from build123d import *

# Parameters (mm, degrees)
SKETCH2_W           = 140
SKETCH2_H           = 140
SKETCH2_R           = 1.6
SKETCH2_R_2         = 1.4
BOSS_EXTRUDE2_DEPTH = 3
SKETCH3_W           = 16
SKETCH3_H           = 3
SKETCH3_W_2         = 3
SKETCH3_H_2         = 16
CUT_EXTRUDE2_DEPTH  = 3


with BuildPart() as part:
    # Sketch2 → Boss-Extrude2 (new body)
    with BuildSketch(Plane(origin=(0, 0, 0), x_dir=(1, 0, 0), z_dir=(0, 1, 0))):
        Rectangle(SKETCH2_W, SKETCH2_H)
        with Locations(Location((-17.011581703, 44.949159058, 0), (0, 0, 270))):
            Circle(SKETCH2_R, mode=Mode.SUBTRACT)
        with Locations(Location((-18.611581703, -3.350840942, 0), (0, 0, 270))):
            Circle(SKETCH2_R, mode=Mode.SUBTRACT)
        with Locations(Location((33.788418297, 29.649159058, 0), (0, 0, 270))):
            Circle(SKETCH2_R, mode=Mode.SUBTRACT)
        with Locations(Location((33.788418297, 1.749159058, 0), (0, 0, 270))):
            Circle(SKETCH2_R, mode=Mode.SUBTRACT)
        with Locations(Location((0, 60, 0), (0, 0, 270))):
            Circle(SKETCH2_R, mode=Mode.SUBTRACT)
        with Locations(Location((-60, 0, 0), (0, 0, 270))):
            Circle(SKETCH2_R, mode=Mode.SUBTRACT)
        with Locations(Location((0, -60, 0), (0, 0, 270))):
            Circle(SKETCH2_R, mode=Mode.SUBTRACT)
        with Locations(Location((60, 0, 0), (0, 0, 270))):
            Circle(SKETCH2_R, mode=Mode.SUBTRACT)
        with Locations(Location((-45, 60, 0), (0, 0, 270))):
            Circle(SKETCH2_R, mode=Mode.SUBTRACT)
        with Locations(Location((45, 60, 0), (0, 0, 270))):
            Circle(SKETCH2_R, mode=Mode.SUBTRACT)
        with Locations(Location((-45, -60, 0), (0, 0, 270))):
            Circle(SKETCH2_R, mode=Mode.SUBTRACT)
        with Locations(Location((45, -60, 0), (0, 0, 270))):
            Circle(SKETCH2_R, mode=Mode.SUBTRACT)
        with Locations(Location((-0.030225379, -18.62367845, 0), (0, 0, 270))):
            Circle(SKETCH2_R_2, mode=Mode.SUBTRACT)
        with Locations(Location((-13.780225379, -40.12367845, 0), (0, 0, 270))):
            Circle(SKETCH2_R_2, mode=Mode.SUBTRACT)
        with Locations(Location((13.719774621, -40.12367845, 0), (0, 0, 270))):
            Circle(SKETCH2_R_2, mode=Mode.SUBTRACT)
    extrude(amount=BOSS_EXTRUDE2_DEPTH)

    # Sketch3 → Cut-Extrude2 (cut)
    with BuildSketch(Plane(origin=(0, 3, 0), x_dir=(1, 0, 0), z_dir=(0, 1, 0))):
        with Locations((-22.5, 68.5)):
            Rectangle(SKETCH3_W, SKETCH3_H)
        with Locations((-22.5, -68.5)):
            Rectangle(SKETCH3_W, SKETCH3_H)
        with Locations((22.5, -68.5)):
            Rectangle(SKETCH3_W, SKETCH3_H)
        with Locations((22.5, 68.5)):
            Rectangle(SKETCH3_W, SKETCH3_H)
        with Locations((-68.5, 22.5)):
            Rectangle(SKETCH3_W_2, SKETCH3_H_2)
        with Locations((68.5, 22.5)):
            Rectangle(SKETCH3_W_2, SKETCH3_H_2)
        with Locations((68.5, -22.5)):
            Rectangle(SKETCH3_W_2, SKETCH3_H_2)
        with Locations((-68.5, -22.5)):
            Rectangle(SKETCH3_W_2, SKETCH3_H_2)
    extrude(amount=-CUT_EXTRUDE2_DEPTH, mode=Mode.SUBTRACT)


solid = part.part
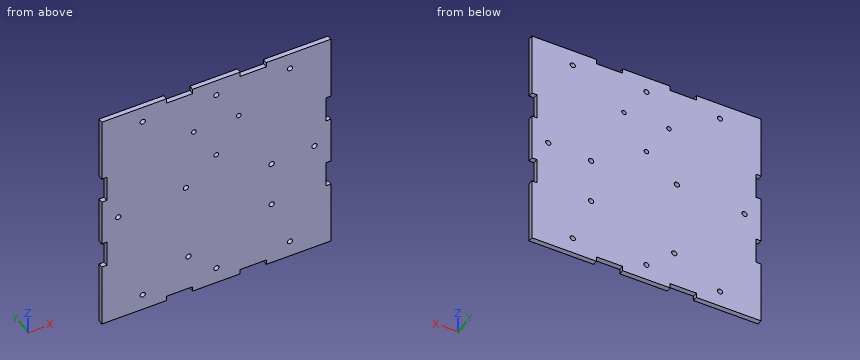
Can you work these out from the model? Positions are in its coordinate system, mm. Coordinates: 2 decimals unless noted, no trailing zeros. Order: outer loops, then holes, each group sorted by start corner. A loop starts at its lowest first (then second) coordinate and runs counter-clockwise, first axis right, second up. Notation, with made-up numbers: (2.5, 3.5) - (46.5, 3.5) arc R20 ccw to (46.5, 23.5) - close; hole circle Ø7 at (-5, 85). An arc over 180 degrees is marked (long way). Answer as a JSON object with one key per item and string values. Group by question number.
Q1. I need wall thicknesses on line 1 (X direction, y = 1.95, z = 60); line 2 (Z direction, x = 33, y = 2.5); line 3 (X direction, y = 1.35, z = 30). Which ranges of each line are inside material? Lowest first, please. Write a range as from..to.
Q2. Imagine slicing it at A-A (x = 60). Please give me the cut outline in (y, z).
Q3. Imagine slicing it at C-C (z = 24.5). Please give me the cut outline in (x, y).
Q4. Imagine slicing it at D-D (y = 1.4). Give the number of separate pieces and of enclosed holes in the cut face, and give its area (3 significant figures).
Q5. Imagine slicing it at B-B (z = -60). Please give me the cut outline in (x, y).
Q6. Will this pin go through, and if not, where does the flat tip stop? P1, Ø1.5, axis at x = 19, y = 1.5, coming from the +Z side.
Determined:
{
 "1": {"line 1": "x = -70..-46.6, -43.4..-1.6, 1.6..43.4, 46.6..70", "line 2": "z = -70..-31.04, -28.26..-3.14, -0.36..70", "line 3": "x = -67..67"},
 "2": {"outline": "(0, -70) - (3, -70) - (3, -1.6) - (0, -1.6) - close; (0, 1.6) - (3, 1.6) - (3, 70) - (0, 70) - close"},
 "3": {"outline": "(-67, 0) - (67, 0) - (67, 3) - (-67, 3) - close"},
 "4": {"separate pieces": "1", "enclosed holes": "15", "area": "19,100 mm2"},
 "5": {"outline": "(-70, 0) - (-46.6, 0) - (-46.6, 3) - (-70, 3) - close; (-43.4, 0) - (-1.6, 0) - (-1.6, 3) - (-43.4, 3) - close; (1.6, 0) - (43.4, 0) - (43.4, 3) - (1.6, 3) - close; (46.6, 0) - (70, 0) - (70, 3) - (46.6, 3) - close"},
 "6": {"P1": "stops at z = 67"}
}
